from build123d import *

# Parameters (mm, degrees)
F0_W     = 25.4
F0_H     = 25.4
F1_DEPTH = 28.575
F2_W     = 7.9375
F2_H     = 1.5875
F3_DEPTH = 11.1125
F4_R     = 2.38125
F5_DEPTH = 12.954
F6_R     = 5.08
F7_SIZE  = 2.54
F8_W     = 4.7625
F8_H     = 12.7
F9_DEPTH = 12.7


with BuildPart() as f1:
    # F0 (on Top) → F1 (new body)
    with BuildSketch(Plane.XY):
        with Locations((-12.7, 12.7)):
            Rectangle(F0_W, F0_H)
    extrude(amount=F1_DEPTH)

    # F2 (on face) → F3 (join)
    with BuildSketch(Plane.XY.offset(28.575)):
        with Locations((-11.90625, 7.14375)):
            Rectangle(F2_W, F2_H)
        with Locations((-11.90625, 18.25625)):
            Rectangle(F2_W, F2_H)
    extrude(amount=F3_DEPTH)

    # F4 (on face) → F5 (cut)
    with BuildSketch(Plane.XZ.offset(-6.35)):
        with Locations((-11.90625, 34.925)):
            Circle(F4_R)
    extrude(amount=-F5_DEPTH, mode=Mode.SUBTRACT)

    # F6
    f6_edges = [f1.edges().sort_by_distance(p)[0] for p in [
        (0, 25.4, 14.2875),
        (0, 0, 14.2875),
        (-25.4, 0, 14.2875),
        (-25.4, 25.4, 14.2875),
    ]]
    fillet(f6_edges, radius=F6_R)

    # F7
    f7_edges = [f1.edges().sort_by_distance(p)[0] for p in [
        (-15.875, 18.25625, 39.6875),
        (-7.9375, 18.25625, 39.6875),
        (-7.9375, 7.14375, 39.6875),
        (-15.875, 7.14375, 39.6875),
    ]]
    chamfer(f7_edges, length=F7_SIZE)

    # F8 (on face) → F9 (cut)
    with BuildSketch(Plane(origin=(0, 0, 0), x_dir=(1, 0, 0), z_dir=(0, 0, -1))):
        with Locations((-8.73125, -12.7)):
            Rectangle(F8_W, F8_H)
    extrude(amount=-F9_DEPTH, mode=Mode.SUBTRACT)


solid = f1.part
Work out the finished part from the listing and answer in its coordinate system (mm). A direction names the side the tool comes from. Give positions to 0.01 mm unless a question says otherwise; leave off trailing zeros. Write each loop counter-clockwise with the first axis right and the second up, starting at its lowest first coordinate (ties: lowest second). Pieces come first, ordered by that corner, then holes. Notation, with made-up numbers: (25, 41) - (61, 41) arc R12 ccw to (61, 51) - close; hole circle Ø7 at (79, 36.5). An arc over 180 degrees is marked (long way). One line per item, written item: value. Start each with the question number.
1. For a pull along Y with two mould halves and no side action, classify faces 1 (the flat face through (-9, 13, 12.7)), 2 (the cylindrical face through (-23.951, 1.528, 14.488)), 3 (the flat face through (0, 13, 14)) as +Y half, -Y half, draft (parallel to the pull), parting line (faces both ways), or undercut.
2. For faces 4 (the flat face through (-7.938, 18, 33)), 5 (the flat face through (-9, 19.05, 6)), 6 (the flat face through (-12, 19.05, 32)), 7 (the flat face through (-15.875, 7, 33)), 8 (the flat face through (-12, 6.35, 32)), determine the directions among +Z, -Z, +X, -X, +Y, -Y from which every point of the face is accessible in a straight line to the end or side of a thin tool.
3. Consider probe 1 along X at (y, z) = (18.5, 5); probe 2 along Y at (x, z) = (-8.75, 37); probe 3 along Z at (x, y) = (-13.5, 10) (3 decimals). Determine where each line is inside the solid, lowest interval first.
4. Find section A-A (z = 3). Write down the section's boundary in (x, y), then the cut area to 3 significant figures.
5. Find section C-C (z = 26.5). Write down the section's boundary in (x, y).
6. Given pin 1 (6 mm diameter, centred on x = -11.91, z = 34.92, fed in from -Y); pin 2 (5 mm diameter, centred on x = -6.5, y = 9, fed in from +Z); pin 3 (1.3 mm diameter, centred on y = 18, z = 32, fed in from -X) (3 decimals); pin 4 (3 mm diameter, centred on x = -11.91, z = 34.92, fed in from +Y), each flat-ended and moving along its own axis, determine where each tip first touches the part or whether it passes through.
Geometry results:
1. face 1: undercut
1. face 2: -Y half
1. face 3: draft
2. face 4: +Z, +X, +Y, -Y
2. face 5: -Z
2. face 6: +Z, +X, -X, +Y
2. face 7: +Z, -X, +Y, -Y
2. face 8: +Z, +X, -X, -Y
3. probe 1: -25.4 to -11.11, -6.35 to 0
3. probe 2: 6.35 to 7.94, 17.46 to 19.05
3. probe 3: 0 to 28.575
4. outline: (-25.4, 5.08) arc R5.08 ccw to (-20.32, 0) - (-5.08, 0) arc R5.08 ccw to (0, 5.08) - (0, 20.32) arc R5.08 ccw to (-5.08, 25.4) - (-20.32, 25.4) arc R5.08 ccw to (-25.4, 20.32) - close; hole (-11.11, 6.35) - (-6.35, 6.35) - (-6.35, 19.05) - (-11.11, 19.05) - close
4. area: 563 mm2
5. outline: (-25.4, 5.08) arc R5.08 ccw to (-20.32, 0) - (-5.08, 0) arc R5.08 ccw to (0, 5.08) - (0, 20.32) arc R5.08 ccw to (-5.08, 25.4) - (-20.32, 25.4) arc R5.08 ccw to (-25.4, 20.32) - close
6. pin 1: y = 6.35
6. pin 2: z = 37.97
6. pin 3: x = -15.875
6. pin 4: through
